Geometry: final body of the model. Coordinates: model frame, mm. Coordinates: 2 decimals unless noted, no trailing zeros. Write each loop counter-clockwise with the first axis right and the second up, starting at its lowest first coordinate (ties: lowest second). Pieces come first, ordered by that corner, then holes. Notation, with made-up numbers: M -27.5,42.25 L -22.5,42.25 A20 cw -22.5,73.25 Z; hole C 34.5,-6.5 d6. An arc over 180 degrees is marked long. Write item = value, one per line. Start each with the question number.
Item 1: Section A-A on y = 1.4. Output: boundary loops of the cut face in (x, z), plus the area to 3 significant figures.
Item 2: Ray query, L1, parallel to Z at x = -19.5, y = 0.85; L2, parallel to X at y = 0.5, z = 19; L3, parallel to X at y = 0.75, z = -18. Return the intervals inside material, ascending. Write a range as [from, to].
Item 3: Section B-B on x = 18.5. Give the number of separate pieces and of enclosed holes in the cut face, plus the area to 3 significant figures.
Item 4: Pull-direction query (Z, two-part tool) for faces 1 (the conical face through (18.73, 1.68, 18.34)), 2 (the flat face through (0, 1, -25)), 3 (the flat face through (0, 0, 0)); classes: +Z half, -Z half, draft (parallel to the pull), parting line (faces both ways), or undercut.
from build123d import *

# Parameters (mm, degrees)
SKETCH1_W           = 50
SKETCH1_H           = 50
BOSS_EXTRUDE1_DEPTH = 2
FILLET2_R           = 10
HOLE1_D             = 3.6
HOLE1_DEPTH         = 10
HOLE1_CSINK_D       = 7.1
HOLE1_CSINK_ANGLE   = 82


with BuildPart() as part:
    # Sketch1 → Boss-Extrude1 (new body)
    with BuildSketch(Plane(origin=(0, 0, 0), x_dir=(1, 0, 0), z_dir=(0, 1, 0))):
        Rectangle(SKETCH1_W, SKETCH1_H)
    extrude(amount=BOSS_EXTRUDE1_DEPTH)

    # Fillet2
    fillet2_edges = [part.edges().sort_by_distance(p)[0] for p in [
        (25, 1, 25),
        (-25, 1, 25),
        (-25, 1, -25),
        (25, 1, -25),
    ]]
    fillet(fillet2_edges, radius=FILLET2_R)

    # Hole1
    with Locations(Plane(origin=(-20, 0, 20), x_dir=(0, 0, -1), z_dir=(0, -1, 0))):
        with Locations((0, 0), (0, 40), (40, 40), (40, 0)):
            CounterSinkHole(HOLE1_D / 2, HOLE1_CSINK_D / 2, depth=HOLE1_DEPTH, counter_sink_angle=HOLE1_CSINK_ANGLE)


solid = part.part
Responses:
q1.outline = M -25,-15 A10 ccw -15,-25 L 15,-25 A10 ccw 25,-15 L 25,15 A10 ccw 15,25 L -15,25 A10 ccw -25,15 Z; hole C -20,-20 d4.67; hole C -20,20 d4.67; hole C 20,-20 d4.67; hole C 20,20 d4.67
q1.area = 2,350 mm²
q2.L1 = [-23.93, -22.77], [-17.23, 17.23], [22.77, 23.93]
q2.L2 = [-24.17, -22.95], [-17.05, 17.05], [22.95, 24.17]
q2.L3 = [-24.54, -22.1], [-17.9, 17.9], [22.1, 24.54]
q3.separate_pieces = 3
q3.enclosed_holes = 0
q3.area = 79.9 mm²
q4.face_1 = undercut
q4.face_2 = -Z half
q4.face_3 = draft
